```python
from build123d import *

# Parameters (mm, degrees)
PAD_DEPTH       = 20
SKETCH001_R     = 4.5
POCKET_DEPTH    = 5
SKETCH002_R     = 3.25
POCKET001_DEPTH = 5


with BuildPart() as part:
    # Sketch → Pad (new body)
    with BuildSketch(Plane.XY):
        with BuildLine():
            Line((0, 28.5), (0, 1.5))
            ThreePointArc((0, 1.5), (0.43934, 0.43934), (1.5, 0))
            Line((1.5, 0), (25, 0))
            ThreePointArc((25, 0), (26.06066, 0.43934), (26.5, 1.5))
            Line((26.5, 1.5), (26.5, 3.5))
            ThreePointArc((26.5, 3.5), (26.06066, 4.56066), (25, 5))
            Line((25, 5), (7, 5))
            ThreePointArc((5, 7), (5.585786, 5.585786), (7, 5))
            Line((5, 7), (5, 28.5))
            ThreePointArc((5, 28.5), (4.56066, 29.56066), (3.5, 30))
            Line((3.5, 30), (1.5, 30))
            ThreePointArc((1.5, 30), (0.43934, 29.56066), (0, 28.5))
        make_face()
    extrude(amount=PAD_DEPTH)

    # Sketch001 (on Face1 of Pad) → Pocket (cut)
    with BuildSketch(Plane.YZ.offset(5)):
        with Locations((15, 10)):
            Circle(SKETCH001_R)
    extrude(amount=-POCKET_DEPTH, mode=Mode.SUBTRACT)

    # Sketch002 (on Face7 of Pocket) → Pocket001 (cut)
    with BuildSketch(Plane(origin=(0, 5, 0), x_dir=(-1, 0, 0), z_dir=(0, 1, 0))):
        with Locations((-15, 10)):
            Circle(SKETCH002_R)
    extrude(amount=-POCKET001_DEPTH, mode=Mode.SUBTRACT)


solid = part.part
```
Design review of the part built by this model. Coordinates are the model's own, in mm. A direction names the side the tool comes from. Coordinates: 2 decimals unless noted, no trailing zeros. Loops run counter-clockwise (first coordinate to the right, second up) from the corner with the lowest first, then second, coordinate; pieces in that order, holes last. Notation, with made-up numbers: (7.5, 35) - (29.5, 35) arc R17 ccw to (29.5, 62) - close; hole circle Ø1 at (21.5, 89.5). An arc over 180 degrees is marked (long way). Use CSV: the item, a comma, the result in double quotes. Start each with the question number.
1) Wall thickness on L1, parallel to Z at x = 15, y = 2.25; L2, parallel to Z at x = 3.15, y = 15; L3, parallel to Y at x = 8.75, z = 19: over which ranges is each line inside the solid? List them lowest first. Write a range as from..to.
2) Consider section D-D on z = 16.5. Write out the cut boundary in (x, y), then the cut area to 3 significant figures.
3) Consider section A-A on x = 15. Write out the cut boundary in (y, z).
4) Consider section B-B on z = 10. Write out the cut boundary in (x, y), then the cut area to 3 significant figures.
5) Consider section C-C on y = 15. Write out the cut boundary in (x, z).
6) For pin 1 Ø4 at (y, z) = (26, 2) entering from +X; pin 2 Ø1 at (x, z) = (7.5, 14.5) entering from -Y; pin 3 Ø10 at (x, z) = (23.5, 2) entering from +Y, all flat-tipped, find the tip position at first contact; note any pin that passes through.
7) The part is to be moulded in two halves that separate along X. For faces 1 (the flat face through (5, 20, 10)), 2 (the flat face through (3, 30, 10)), 3 (the cylindrical face through (17.395, 2.535, 12.197)), 4 (the flat face through (0, 15, 5)), say which applies: +X half, -X half, draft (parallel to the pull), parting line (faces both ways), or undercut.
8) Tool access review of faces 5 (the cylindrical face through (0.45, 29.57, 9.86)), 6 (the flat face through (18, 5, 8)): name each direction out of +Z, -Z, +X, -X, +Y, -Y from which nothing blocks a thin tool from reaching the whole face with its end or side.
Geometry says:
1,L1,"0..6.75, 13.25..20"
1,L2,"0..5.5, 14.5..20"
1,L3,"0..5"
2,outline,"(0, 1.5) arc R1.5 ccw to (1.5, 0) - (25, 0) arc R1.5 ccw to (26.5, 1.5) - (26.5, 3.5) arc R1.5 ccw to (25, 5) - (7, 5) arc R2 cw to (5, 7) - (5, 28.5) arc R1.5 ccw to (3.5, 30) - (1.5, 30) arc R1.5 ccw to (0, 28.5) - close"
2,area,"256 mm^2"
3,outline,"(0, 0) - (5, 0) - (5, 6.75) - (0, 6.75) - close; (0, 13.25) - (5, 13.25) - (5, 20) - (0, 20) - close"
4,outline,"(0, 1.5) arc R1.5 ccw to (1.5, 0) - (11.75, 0) - (11.75, 5) - (7, 5) arc R2 cw to (5, 7) - (5, 10.5) - (0, 10.5) - close; (0, 19.5) - (5, 19.5) - (5, 28.5) arc R1.5 ccw to (3.5, 30) - (1.5, 30) arc R1.5 ccw to (0, 28.5) - close; (18.25, 0) - (25, 0) arc R1.5 ccw to (26.5, 1.5) - (26.5, 3.5) arc R1.5 ccw to (25, 5) - (18.25, 5) - close"
4,area,"178 mm^2"
5,outline,"(0, 0) - (5, 0) - (5, 5.5) - (0, 5.5) - close; (0, 14.5) - (5, 14.5) - (5, 20) - (0, 20) - close"
6,pin 1,"x = 5"
6,pin 2,"y = 0"
6,pin 3,"y = 5"
7,face 1,"+X half"
7,face 2,"draft"
7,face 3,"undercut"
7,face 4,"-X half"
8,face 5,"+Z, -Z, -X, +Y"
8,face 6,"+Z, -Z, +X, +Y"
